Autodesk Inventor part; units mm, degrees
ref_plane "YZ Plane" through (0, 0, 0) normal (1, 0, 0) x (0, 1, 0)
ref_plane "XZ Plane" through (0, 0, 0) normal (0, 1, 0) x (-1, 0, 0)
ref_plane "XY Plane" through (0, 0, 0) normal (0, 0, 1) x (1, 0, 0)
sketch "Sketch1" plane through (0, 0, 0) normal (0, 0, 1) x (1, 0, 0)
  line L0 (0, 0) -> (0, 137.0131)
  line L1 (-11.7886, 12.2907) -> (-39.6863, 18.4755) construction
  line L2 (-39.6863, 18.4755) -> (-33.3297, 47.1481) construction
  line L3 (-33.3297, 47.1481) -> (-5.432, 40.9633) construction
  line L4 (-5.432, 40.9633) -> (-11.7886, 12.2907) construction
  line L5 (-39.6863, 18.4755) -> (-5.432, 40.9633) construction
  line L6 (-33.3297, 47.1481) -> (-11.7886, 12.2907) construction
  circle A0 centre (-53.975, 12.7) radius 3.175
  circle A1 centre (-53.975, 12.7) radius 9.525
  line L7 (0, 0) -> (-54.5315, 3.1913) construction
  line L8 (-62.4238, 17.0982) -> (0, 137.0131)
  line L9 (-27.1302, 45.7737) -> (-37.4529, 28.5497) construction
  line L10 (-11.6315, 42.3377) -> (-9.5552, 22.3649) construction
  line L11 (-19.3809, 44.0557) -> (-25.7374, 15.3831) construction
  line L12 (0, 104.775) -> (-15.0457, 108.1106)
  line L13 (-35.3766, 8.5768) -> (-19.8779, 5.1408) construction
  line L14 (-19.8779, 5.1408) -> (-21.2523, -1.0586) construction
  line L15 (-21.2523, -1.0586) -> (-36.751, 2.3773) construction
  line L16 (-36.751, 2.3773) -> (-35.3766, 8.5768) construction
  line L17 (-35.3766, 8.5768) -> (-44.7305, 2.6177) construction
  line L18 (-19.8779, 5.1408) -> (-17.2457, 1.0092) construction
  line L19 (-5.432, 40.9633) -> (-33.3297, 47.1481) construction
  line L20 (-33.3297, 47.1481) -> (-32.2475, 52.0296) construction
  line L21 (-32.2475, 52.0296) -> (-4.3498, 45.8448) construction
  line L22 (-4.3498, 45.8448) -> (-5.432, 40.9633) construction
  line L23 (-53.2878, 15.7997) -> (-53.975, 12.7) construction
  line L24 (-53.975, 12.7) -> (-57.0747, 13.3872) construction
  line L25 (-27.6272, 6.8588) -> (-34.4992, -24.1386) construction
  line L26 (-31.8676, 50.076) -> (-5.5198, 44.2349) construction
  line L27 (-5.5198, 44.2349) -> (-4.489, 48.8845) construction
  line L28 (-4.489, 48.8845) -> (-30.8368, 54.7256) construction
  line L29 (-30.8368, 54.7256) -> (-31.8676, 50.076) construction
  line L30 (-31.3522, 52.4008) -> (-5.0044, 46.5597) construction
  circle A2 centre (-29.0274, 51.8854) radius 1.4732 construction
  circle A3 centre (-22.8279, 50.5111) radius 1.4732 construction
  circle A4 centre (-16.6284, 49.1367) radius 1.4732
  circle A5 centre (-10.4289, 47.7623) radius 1.4732
  circle A6 centre (-7.6985, 96.7513) radius 1.4732
  line L31 (-53.975, 12.7) -> (-5.4185, 105.9762)
  line L32 (-31.2085, 56.4341) -> (0, 49.5153)
  circle A7 centre (-7.6985, 96.7513) radius 4.7625
  line L33 (-4.7625, 50.5712) -> (-4.7625, 105.8308)
  line L34 (-26.3948, 55.3669) -> (-7.323, 92.0036)
  line L35 (-3.5958, 94.3328) -> (-4.7625, 94.5914) construction
  line L36 (-17.2457, 1.0092) -> (0, 1.0092) construction
  line L37 (0, 1.0092) -> (0, -2.1658) construction
  line L38 (0, -2.1658) -> (-17.2457, -2.1658) construction
  line L39 (-17.2457, -2.1658) -> (-17.2457, 1.0092) construction
  circle A8 centre (-12.7, 7.9375) radius 1.5875 construction
  line L40 (-12.7, 7.9375) -> (0, 7.9375) construction
  line L41 (0, 7.9375) -> (-17.2457, 1.0092)
  circle A9 centre (-12.7, 7.9375) radius 3.175 construction
  line L42 (-9.525, 7.9375) -> (-9.525, 4.111) construction
  line L43 (-9.525, 7.9375) -> (0, 7.9375) construction
  line L44 (-17.9187, 46.9837) -> (-16.8879, 51.6333) construction
  line L45 (-12.4942, 45.7811) -> (-26.2381, -16.2137) construction
  line L46 (0, 53.6985) -> (0, 7.9375) construction
  line L47 (-26.2381, -16.2137) -> (-20.0386, -17.5881) construction
  line L48 (-20.0386, -17.5881) -> (-8.7313, 7.9375)
  circle A10 centre (-12.7, 6.35) radius 1.4224
  line L49 (0, 13.4938) -> (-4.7625, 13.4938) construction
  line L50 (-4.7625, 13.4938) -> (-4.7625, 24.6063) construction
  line L51 (-4.7625, 24.6063) -> (0, 24.6063) construction
  line L52 (0, 24.6063) -> (0, 13.4938) construction
  line L53 (-4.7625, 19.05) -> (0, 19.05) construction
  circle A11 centre (-2.3813, 19.05) radius 1.4224
  line L54 (-20.7405, 8.5842) -> (-9.7454, 58.18) construction
  line L55 (-9.7454, 58.18) -> (-3.5459, 56.8056) construction
  line L56 (-3.5459, 56.8056) -> (-14.5411, 7.2098) construction
  line L57 (-14.5411, 7.2098) -> (-20.7405, 8.5842) construction
  line L58 (-12.7, 6.35) -> (-12.7, 7.9375) construction
  line L59 (-11.5442, 1.5875) -> (-9.525, 1.5875) construction
  line L60 (-9.525, 1.5875) -> (-9.525, 7.9375) construction
  line L61 (-9.525, 7.9375) -> (-11.5442, 7.9375) construction
  line L62 (-11.5442, 7.9375) -> (-11.5442, 1.5875) construction
  line L63 (-9.7454, 58.18) -> (-15.9449, 59.5544) construction
  line L64 (-18.8691, 53.6985) -> (0, 53.6985)
  line L65 (-9.7454, 58.18) -> (-17.3193, 53.3549) construction
  arc A12 (-10.2313, 55.9882) -> (-11.9373, 58.6659) centre (-11.0843, 57.3271) ccw construction
  line L66 (-4.7625, 57.15) -> (0, 57.15) construction
  circle A13 centre (-2.3813, 57.15) radius 1.4224
  circle A14 centre (-2.3813, 63.5) radius 1.4224
  line L67 (0, 7.9375) -> (-38.5755, 7.9375) construction
  line L68 (-38.5755, 7.9375) -> (-38.5755, -42.8625) construction
  line L69 (-38.5755, -42.8625) -> (0, -42.8625)
  line L70 (0, -42.8625) -> (0, 7.9375)
  line L71 (-38.5755, -42.8625) -> (-62.6076, 8.6746)
  line L72 (-60.0032, 20.0747) -> (-18.8691, 53.6985)
  line L73 (-20.0386, -17.5881) -> (-20.0386, -42.8625) construction
  line L74 (-20.2435, 47.4991) -> (-19.2127, 52.1487) construction
  line L75 (-12.7, -42.8625) -> (-12.7, -1.0217)
  circle A15 centre (-23.8125, -33.3375) radius 1.7526
  circle A16 centre (-15.875, -28.575) radius 1.7526
  circle A17 centre (-23.8125, -33.3375) radius 3.175 construction
  circle A18 centre (-2.3813, 69.85) radius 1.4224
  circle A19 centre (-2.3813, 76.2) radius 1.4224
  circle A20 centre (-15.875, -28.575) radius 3.175 construction
  circle A21 centre (-46.0375, -19.05) radius 1.7526
  arc A22 (0, 104.775) -> (-15.0457, 108.1106) centre (-7.9697, 104.427) ccw
  circle A23 centre (-7.9697, 104.427) radius 1.4224
  line L76 (-7.9697, 104.427) -> (-15.0457, 108.1106) construction
  line L77 (-7.9697, 104.427) -> (0, 104.775) construction
  line L78 (-14.2148, 89.0787) -> (-22.6636, 93.4768)
  point P0 (-22.5591, 29.7194)
  point P1 (-20.7484, 1.2142)
  point P2 (-36.3367, 4.2458)
  point P3 (-49.5768, 21.1488)
  point P4 (-11.1125, 7.9375)
  point P5 (-11.4283, 6.9872)
  point P6 (-11.9574, 7.9375)
  point P7 (-13.9717, 6.9872)
  point P8 (-9.525, 6.1457)
  point P9 (-10.6215, 3.6705)
  point P10 (-4.7625, 93.0015)
  point P11 (-4.7625, 53.6985)
  dimension "d74" = 6.35
  dimension "d14" = 29.3687
  dimension "d15" = 28.575
  dimension "d16" = 12.5
  dimension "d17" = 6.35
  dimension "d19" = 53.975
  dimension "d22" = 19.05
  dimension "d23" = 7.9375
  dimension "d24" = 19.05
  dimension "d26" = 102.5
  dimension "d29" = 6.35
  dimension "d31" = 7.9375
  dimension "d34" = 5
  dimension "d35" = 26.9875
  dimension "d38" = 31.75
  dimension "d40" = 26.9875
  dimension "d41" = 4.7625
  dimension "d42" = 2.9464
  dimension "d43" = 2.3813
  dimension "d46" = 6.35
  dimension "d51" = 2.9464
  dimension "d52" = 92.075
  dimension "d53" = 6.35
  dimension "d54" = 9.525
  dimension "d55" = 4.7625
  dimension "d56" = 4.7625
  dimension "d60" = 12.7
  dimension "d61" = 3.175
  dimension "d63" = 3.175
  dimension "d66" = 3.175
  dimension "d67" = 12.7
  dimension "d72" = 8.7312
  dimension "d73" = 7.9375
  dimension "d80" = 12.7
  dimension "d82" = 7.9375
  dimension "d83" = 63.5
  dimension "d85" = 6.35
  dimension "d86" = 104.775
  dimension "d87" = 2.8448
  dimension "d88" = 4.7625
  dimension "d89" = 11.1125
  dimension "d90" = 2.8448
  dimension "d91" = 19.05
  dimension "d92" = 6.35
  dimension "d93" = 50.8
  dimension "d94" = 25.4
  dimension "d95" = 8.7312
  dimension "d96" = 9.525
  dimension "d97" = 6.35
  dimension "d99" = 6.35
  dimension "d101" = 3.175
  dimension "d106" = 2.8448
  dimension "d107" = 57.15
  dimension "d110" = 6.35
  dimension "d136" = 3.175
  dimension "d138" = 42.8625
  dimension "d139" = 12.7
  dimension "d140" = 3.5052
  dimension "d141" = 3.5052
  dimension "d142" = 9.525
  dimension "d143" = 3.175
  dimension "d144" = 11.1125
  dimension "d145" = 6.35
  dimension "d146" = 14.2875
  dimension "d149" = 6.35
extrude "Extrusion1" add sketch "Sketch1" along normal blind 3.175 contours L41 L48 L75 L69 L71 A1 L31 L72 L32 L0 | L32 L33 L64 L0 | L64 L33 A7 L12 L0 | L32 L64 L33 | L12 A22 | L72 L31 L32 | A1 | L33 A7 L31 L12 | L12 L31 A7 L78 L8 | L33 A7 | A7 L31 L33 | L32 L31 A7 L34 | L31 A7
fillet "Fillet6" radius 12.7 1 edges at (-38.5755, -42.8625, 1.5875)
fillet "Fillet7" radius 6.35 3 edges at (-22.6636, 93.4768, 1.5875) (-14.2148, 89.0787, 1.5875) (-49.5768, 21.1488, 1.5875)
fillet "Fillet8" radius 4.7625 5 edges at (-4.7625, 93.0015, 1.5875) (-7.323, 92.0036, 1.5875) (-26.3948, 55.3669, 1.5875) (-18.8691, 53.6985, 1.5875) (-4.7625, 53.6985, 1.5875)
fillet "Fillet9" radius 9.525 3 edges at (-10.6215, 3.6705, 1.5875) (-12.7, -1.0217, 1.5875) (-12.7, -42.8625, 1.5875)
equation "\"d56\" = d55"
properties part number "Uprights" material "UHMW, White"
Verification items for the finished model (mm, model axes). A direction names the side the tool comes from. Give positions to 0.01 mm unless a question says otherwise; leave off trailing zeros. Write each loop counter-clockwise with the first axis right and the second up, starting at its lowest first coordinate (ties: lowest second). Pieces come first, ordered by that corner, then holes.
(1) Cross-section at D-D (y = -19.05). Enter the section's corners in (x, z) (3 decimals).
(2) Material ranges on line 1 (X direction, y = 76, z = 2.5); line 2 (Y direction, x = -3, z = 1.9); line 3 (Y direction, x = -15, z = 2.1), recorded low to high.
(3) Access from +Z, -Z, +X, -X, +Y, -Y to the whole of each face (thin tool, end or side, straight path). Record for faces 1 (the face through (-25, 19, 3.175)), 2 (the face through (-18.707, 70.136, 1.565)).
(4) Gauge pin test, flat ends, axial feed: pin 1 (4.5 mm diameter, centred on x = -46.04, y = -19.05, fed in from +Z) (3 decimals); pin 2 (1.5 mm diameter, centred on x = -12.5, z = 2, fed in from +Y); pin 3 (1.5 mm diameter, centred on x = -30.5, z = 2.5, fed in from +Y); pin 4 (1 mm diameter, centred on x = -12, z = 2.5, fed in from +Y). Record the tip position at first contact, or that the pin passes through.
(5) Cross-section at A-A (y = 12.7). Enter the section's corners in (x, z) (3 decimals), plus the area to 3 significant figures.
(6) Mould release check, pull along Y, two halves, no side actions. Record for faces 3 (the face through (-3.316, 6.605, 1.565)), 4 (the face through (0, 56, 2)), 5 (the face through (-2.57, 74.79, 1.57)): +Y half, -Y half, draft (parallel to the pull), parting line (faces both ways), or undercut.
(7) Cross-section at C-C (x = -39). Enter the section's corners in (y, z) (3 decimals), plus the area to 3 significant figures.
(8) Cross-section at B-B (y = 63.5). Enter the section's corners in (x, z) (1 decimal), plus the area to 3 significant figures.
Worked out:
1. outline: (-49.679, 0) - (-47.79, 0) - (-47.79, 3.175) - (-49.679, 3.175) - close; (-44.285, 0) - (-12.7, 0) - (-12.7, 3.175) - (-44.285, 3.175) - close
2. line 1: x = -21.02 to -15.65, -4.76 to -3.79, -0.97 to 0
2. line 2: y = 6.73 to 17.77, 20.33 to 55.87, 58.43 to 62.22, 64.78 to 68.57, 71.13 to 74.92, 77.48 to 110.67
2. line 3: y = -39.54 to -30.09, -27.06 to 53.7, 77.26 to 108.2
3. face 1: +Z, +X, -X, +Y, -Y
3. face 2: +Z, -Z
4. pin 1: stops at z = 3.175
4. pin 2: stops at y = 111.45
4. pin 3: stops at y = 59.24
4. pin 4: stops at y = 111.58
5. outline: (-63.5, 0) - (-57.15, 0) - (-57.15, 3.175) - (-63.5, 3.175) - close; (-50.8, 0) - (0, 0) - (0, 3.175) - (-50.8, 3.175) - close
5. area: 181 mm2
6. face 3: -Y half
6. face 4: draft
6. face 5: undercut
7. outline: (-39.585, 0) - (41.467, 0) - (41.467, 3.175) - (-39.585, 3.175) - close
7. area: 257 mm2
8. outline: (-27.5, 0) - (-22.2, 0) - (-22.2, 3.2) - (-27.5, 3.2) - close; (-4.8, 0) - (-3.8, 0) - (-3.8, 3.2) - (-4.8, 3.2) - close; (-1, 0) - (0, 0) - (0, 3.2) - (-1, 3.2) - close
8. area: 23.1 mm2
